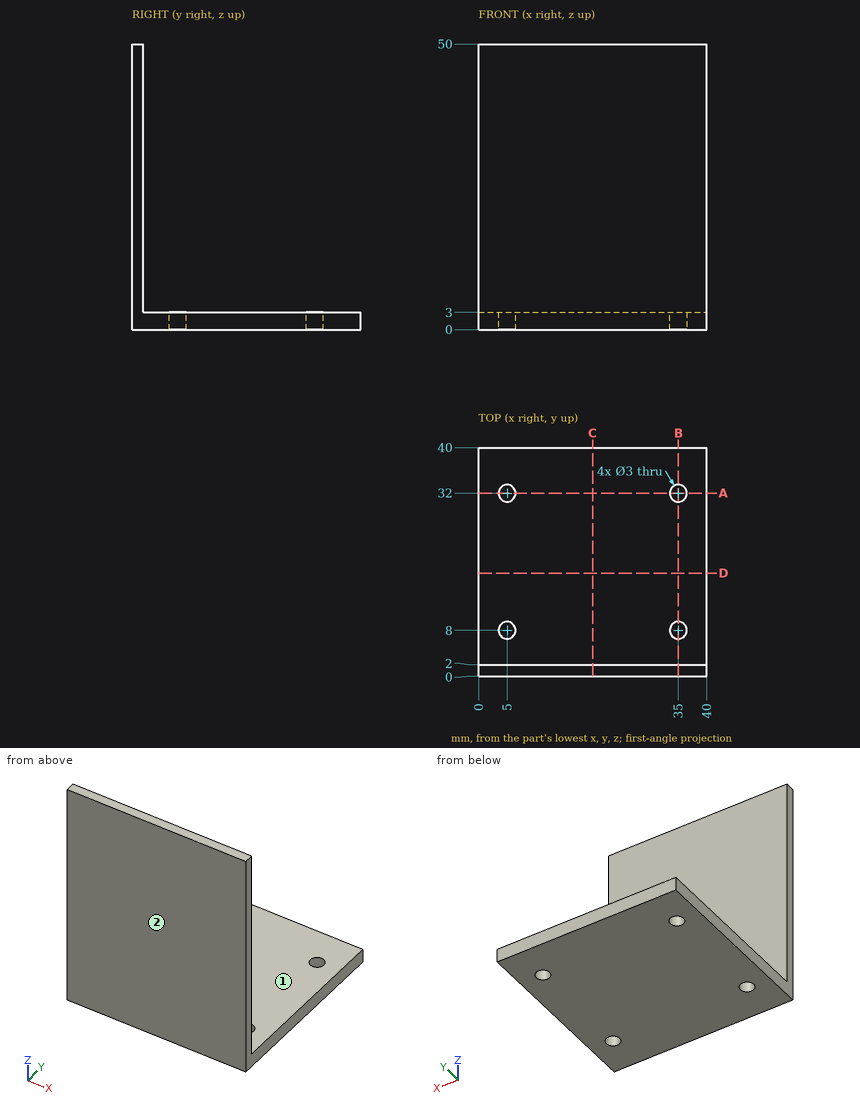
Could you check a few things on this drawing? It's one solid part, dimensions in mm from its lowest x, y, z. A direction names the side the tool comes from. Coordinates: 2 decimals unless noted, no trailing zeros. Order: outer loops, then holes, each group sorted by start corner. A loop starts at its lowest first (then second) coordinate and runs counter-clockwise, first axis right, second up. Notation, with made-up numbers: (65, 72.25) - (79, 72.25) arc R19 ccw to (79, 89.25) - close; hole circle Ø9 at (4, 56.5). An arc over 180 degrees is marked (long way). Answer as a JSON object with one key per item and string values. Group by question number.
Q1. Imagine slicing it at B-B (x = 35). Please give me the cut outline in (y, z), and give its area (3 significant figures).
Q2. Imagine slicing it at A-A (y = 32). Please give me the cut outline in (x, z), and give its area (3 significant figures).
Q3. I need wall thicknesses on line 1 (Y direction, x = 35, z = 1); line 2 (Z direction, x = 17.5, y = 37.5); line 3 (Y direction, x = 21, z = 43.5). Which ranges of each line are inside material? Lowest first, please. Write a range as from..to.
Q4. On a 3-axis mill with a long thin cutter (end or side, diameter ignored), from which of +Z, -Z, +X, -X, +Y, -Y can I reach the whole of each face in a straight line? I mean the marked faces 1 and 2. Say none if no direction works.
Q5. Will these pins go through, and if not, where does the flat tip stop? P1, Ø2.5, axis at x = 5, y = 32, coming from the +Z side; P2, Ø12, axis at x = 11.5, y = 36, coming from the +Z side.
Q6. Imagine slicing it at D-D (y = 18). Please give me the cut outline in (x, z), and give its area (3 significant figures).
Q7. Imagine slicing it at C-C (x = 20). Please give me the cut outline in (y, z).
Determined:
{
 "1": {"outline": "(0, 0) - (6.5, 0) - (6.5, 3) - (2, 3) - (2, 50) - (0, 50) - close; (9.5, 0) - (30.5, 0) - (30.5, 3) - (9.5, 3) - close; (33.5, 0) - (40, 0) - (40, 3) - (33.5, 3) - close", "area": "196 mm2"},
 "2": {"outline": "(0, 0) - (3.5, 0) - (3.5, 3) - (0, 3) - close; (6.5, 0) - (33.5, 0) - (33.5, 3) - (6.5, 3) - close; (36.5, 0) - (40, 0) - (40, 3) - (36.5, 3) - close", "area": "102 mm2"},
 "3": {"line 1": "y = 0..6.5, 9.5..30.5, 33.5..40", "line 2": "z = 0..3", "line 3": "y = 0..2"},
 "4": {"face 1": "+Z, +X, -X, +Y", "face 2": "+Z, -Z, +X, -X, -Y"},
 "5": {"P1": "passes through", "P2": "stops at z = 3"},
 "6": {"outline": "(0, 0) - (40, 0) - (40, 3) - (0, 3) - close", "area": "120 mm2"},
 "7": {"outline": "(0, 0) - (40, 0) - (40, 3) - (2, 3) - (2, 50) - (0, 50) - close"}
}
